CAD build for the part. Positions are in the model's coordinates, mm. Face numbers are marked on the shaded views. Give positions to 0.01 mm unless a question says otherwise; leave off trailing zeros. Write each loop counter-clockwise with the first axis right and the second up, starting at its lowest first coordinate (ties: lowest second). Pieces come first, ordered by that corner, then holes. Notation, with made-up numbers: (60.5, 70.5) - (115.5, 70.5) arc R33 ccw to (115.5, 108.5) - close; hole circle Ø1 at (42, -19). An arc over 180 degrees is marked (long way). Answer as a JSON object with one key per item and string values.
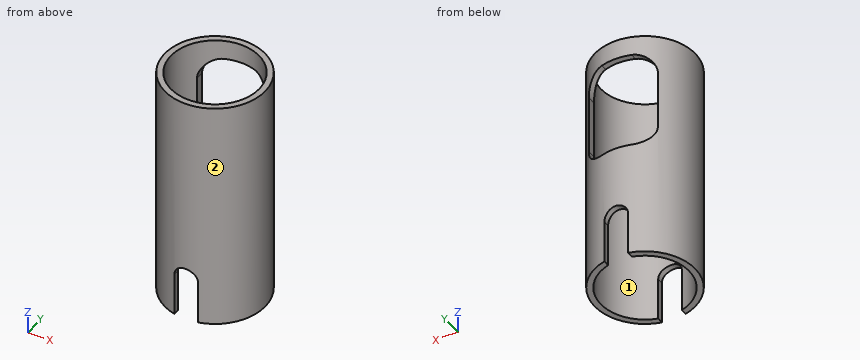
from build123d import *

# Parameters (mm, degrees)
F0_R     = 25.75
F0_R_2   = 22.65
F1_DEPTH = 120
F3_DEPTH = 25.751
F4_DEPTH = 30


with BuildPart() as f1:
    # F0 (on Top) → F1 (new body)
    with BuildSketch(Plane.XY):
        Circle(F0_R)
        Circle(F0_R_2, mode=Mode.SUBTRACT)
    extrude(amount=F1_DEPTH)

    # F2 (on Front) → F3 (cut, through all)
    with BuildSketch(Plane.XZ):
        with BuildLine():
            Line((7.5, 110), (-7.5, 110))
            ThreePointArc((-7.5, 110), (-14.571068, 107.071068), (-17.5, 100))
            Line((-17.5, 100), (-17.5, 70))
            ThreePointArc((-17.5, 70), (-14.571068, 62.928932), (-7.5, 60))
            Line((-7.5, 60), (7.5, 60))
            ThreePointArc((7.5, 60), (14.571068, 62.928932), (17.5, 70))
            Line((17.5, 70), (17.5, 100))
            ThreePointArc((17.5, 100), (14.571068, 107.071068), (7.5, 110))
        make_face()
    extrude(amount=-F3_DEPTH, mode=Mode.SUBTRACT)

    # F2 (on Front) → F4 (cut, symmetric)
    with BuildSketch(Plane.XZ):
        with BuildLine():
            Line((-6, 22), (-6, 0))
            Line((-6, 0), (6, 0))
            Line((6, 0), (6, 22))
            ThreePointArc((6, 22), (0, 28), (-6, 22))
        make_face()
    extrude(amount=F4_DEPTH, both=True, mode=Mode.SUBTRACT)


solid = f1.part
Item 1: Cut at C-C (z = 55). Give the cut face in (x, y), and give its area (3 significant figures).
Entries:
{"outline": "circle Ø51.5 at (0, 0); hole circle Ø45.3 at (0, 0)", "area": "471 mm2"}
Item 2: Mould opens along X. For the marked faces 1 and 2 say: +X half, -X half, draft (parallel to the pull), parting line (faces both ways), or undercut.
Entries:
{"face 1": "undercut", "face 2": "parting line"}
Item 3: Cut at A-A (y = 0). Give the cut face in (x, z).
Entries:
{"outline": "(-25.75, 0) - (-22.65, 0) - (-22.65, 120) - (-25.75, 120) - close; (22.65, 0) - (25.75, 0) - (25.75, 120) - (22.65, 120) - close"}
Item 4: Cut at D-D (x = -20). Give the cut face in (y, z), and give its area (3 significant figures).
Entries:
{"outline": "(-16.22, 0) - (-10.63, 0) - (-10.63, 120) - (-16.22, 120) - close; (10.63, 0) - (16.22, 0) - (16.22, 120) - (10.63, 120) - close", "area": "1,340 mm2"}
Item 5: Flat gauge pins, fed straight in: P1, Ø1.5, axis at y = 10.5, z = 95.5, coming from the +X side; P2, Ø1.4, axis at y = 16.5, z = 80, coming from the +X side; P3, Ø1.6, axis at y = -24, z = 10, coming from the -X side; P4, Ø1, axis at x = -16, y = 14, coming from the -Z side. Where does each tip first touch, or does it go through?
Entries:
{"P1": "x = 23.83", "P2": "x = 20.33", "P3": "x = -11.17", "P4": "through"}
Item 6: Cut at B-B (x = 0). Give the cut face in (y, z).
Entries:
{"outline": "(-25.75, 28) - (-22.65, 28) - (-22.65, 120) - (-25.75, 120) - close; (22.65, 28) - (25.75, 28) - (25.75, 60) - (22.65, 60) - close; (22.65, 110) - (25.75, 110) - (25.75, 120) - (22.65, 120) - close"}
Item 7: Probe line 1 (X direction, y = 0.5, z = 52.5); line 2 (Y direction, x = -12, z = 57); line 3 (Z direction, x = 2, y = 23.5). List the from-to ranges inside material, lowest first. Write a range as from..to.
Entries:
{"line 1": "-25.75..-22.64, 22.64..25.75", "line 2": "-22.78..-19.21, 19.21..22.78", "line 3": "27.66..60, 110..120"}
